```python
from build123d import *

# Parameters (mm, degrees)
F0_W     = 10
F0_H     = 10
F0_W_2   = 32.1
F0_R     = 11.05
F0_R_2   = 7.5
F1_DEPTH = 10
F2_R     = 11.05
F2_R_2   = 7.5
F3_DEPTH = 7
F5_D     = 4.4
F6_R     = 1.5


with BuildPart() as f1:
    # F0 (on Front) → F1 (new body)
    with BuildSketch(Plane.XZ):
        with Locations((-21.05, -22.5)):
            Rectangle(F0_W, F0_H)
        with Locations((0, -22.5)):
            Rectangle(F0_W_2, F0_H)
        with Locations((21.05, -22.5)):
            Rectangle(F0_W, F0_H)
        with BuildLine():
            Line((-16.05, 7.5), (-16.05, -17.5))
            Line((-16.05, -17.5), (16.05, -17.5))
            Line((16.05, -17.5), (16.05, 7.5))
            ThreePointArc((16.05, 7.5), (0, 23.55), (-16.05, 7.5))
        make_face()
        with Locations((0, 7.5)):
            Circle(F0_R, mode=Mode.SUBTRACT)
        with Locations((0, 7.5)):
            Circle(F0_R)
        with Locations((0, 7.5)):
            Circle(F0_R_2, mode=Mode.SUBTRACT)
    extrude(amount=F1_DEPTH)

    # F2 (on face) → F3 (cut)
    with BuildSketch(Plane.XZ.offset(10)):
        with Locations((0, 7.5)):
            Circle(F2_R)
        with Locations((0, 7.5)):
            Circle(F2_R_2, mode=Mode.SUBTRACT)
    extrude(amount=-F3_DEPTH, mode=Mode.SUBTRACT)

    # F5 (through all)
    with Locations(Plane.XY.offset(-17.5)):
        with Locations((-21.05, -5), (21.05, -5)):
            Hole(F5_D / 2)

    # F6
    f6_edges = [f1.edges().sort_by_distance(p)[0] for p in [
        (-16.05, -5, -17.5),
        (-26.05, -5, -17.5),
        (16.05, -5, -17.5),
        (26.05, -5, -17.5),
    ]]
    fillet(f6_edges, radius=F6_R)


solid = f1.part
```
Could you check a few things on this model? Use its own coordinates, in mm. A direction names the side the tool comes from. Round coordinates to 2 decimals unless told otherwise and drop trailing zeros. Order: outer loops, then holes, each group sorted by start corner. A loop starts at its lowest first (then second) coordinate and runs counter-clockwise, first axis right, second up. Notation, with made-up numbers: M -12,41 L -1,41 A25 ccw -1,64 Z; hole C 8,80 d5. An arc over 180 degrees is marked long. One line per question, with ' | ' between items. Start each with the question number.
(1) Thinking about a two-plate mould opening in Y: for faces 1 (the face through (0, 0, -7)), 2 (the face through (-20.2, -2.7, -17.5)), 3 (the face through (22.796, -6.339, -22.57)), which applies, +Y half, -Y half, draft (parallel to the pull), parting line (faces both ways), or undercut?
(2) Suppose I cut it at C-C on z = 11.5. List the corners of the cut face in (x, y) for me.
(3) Please list where these lines run through material, in increasing order: line 1 along Y through (x, z) = (21, -23); line 2 along Z through (x, y) = (18.5, -1); line 3 along Z through (x, y) = (-0.5, -6.25).
(4) Suppose I cut it at B-B on x = -21. List the corners of the cut face in (y, z) for me.
(5) Suppose I cut it at D-D on y = -1. List the corners of the cut face in (x, z) for me.
(6) Suppose I cut it at A-A on y = -5. List the corners of the cut face in (x, z) for me.
(7) For faces 4 (the face through (21.9, -2.7, -17.5)), 5 (the face through (-16.05, -5, -4)), 6 (the face through (-1.438, -6.549, 18.456)), which set-ups out of +Z, -Z, +X, -X, +Y, -Y let a thin tool reach every point of the face, with its end or its side?
(8) For P1, Ø3, axis at y = -4, z = -14, coming from the +X side; P2, Ø9, axis at x = 0, z = 7.5, coming from the +Y side; P3, Ø5, axis at x = 4.5, y = -8.5, coming from the +Z side; P4, Ø1, axis at x = 5, z = -0.5, coming from the +Y side, each with a flat end and sliding along its axis, tell me the tip position at first contact or that it passes through.
Geometry results:
1) face 1: +Y half | face 2: draft | face 3: undercut
2) outline: M -15.54,-10 L -10.3,-10 L -10.3,-3 L -6.34,-3 L -6.34,0 L -15.54,0 Z; M 6.34,-3 L 10.3,-3 L 10.3,-10 L 15.54,-10 L 15.54,0 L 6.34,0 Z
3) line 1: -10 to -7.2, -2.8 to 0 | line 2: -27.5 to -17.5 | line 3: -27.5 to -3.54, 18.54 to 23.54
4) outline: M -10,-27.5 L -7.2,-27.5 L -7.2,-17.5 L -10,-17.5 Z; M -2.8,-27.5 L 0,-27.5 L 0,-17.5 L -2.8,-17.5 Z
5) outline: M -26.05,-27.5 L 26.05,-27.5 L 26.05,-19 A1.5 ccw 24.55,-17.5 L 17.55,-17.5 A1.5 cw 16.05,-16 L 16.05,7.5 A16.05 ccw -16.05,7.5 L -16.05,-16 A1.5 cw -17.55,-17.5 L -24.55,-17.5 A1.5 ccw -26.05,-19 Z; hole C 0,7.5 d15
6) outline: M -26.05,-27.5 L -23.25,-27.5 L -23.25,-17.5 L -24.55,-17.5 A1.5 ccw -26.05,-19 Z; M -18.85,-27.5 L 18.85,-27.5 L 18.85,-17.5 L 17.55,-17.5 A1.5 cw 16.05,-16 L 16.05,7.5 A16.05 ccw -16.05,7.5 L -16.05,-16 A1.5 cw -17.55,-17.5 L -18.85,-17.5 Z; M 23.25,-27.5 L 26.05,-27.5 L 26.05,-19 A1.5 ccw 24.55,-17.5 L 23.25,-17.5 Z; hole C 0,7.5 d22.1
7) face 4: +Z, +X, +Y, -Y | face 5: +Z, -X, +Y, -Y | face 6: -Y
8) P1: x = 16.05 | P2: through | P3: z = 23.42 | P4: y = 0
